from build123d import *

# Parameters (mm, degrees)
SKETCH002_R  = 1
PAD002_DEPTH = 30
PAD_DEPTH    = 6
PAD001_DEPTH = 2
SKETCH003_W  = 5
SKETCH003_H  = 5
POCKET_DEPTH = 0.5


with BuildPart() as screw_hole:
    # Sketch002 → Pad002 (new body)
    with BuildSketch(Plane.XY):
        with Locations((10, 0)):
            Circle(SKETCH002_R)
    extrude(amount=PAD002_DEPTH)


with BuildPart() as pocket:
    # Sketch → Pad (new body)
    with BuildSketch(Plane.XY):
        Polygon((0, 8.5), (8.5, 8.5), (8.5, 2.5), (11.8, 2.5), (11.8, -2.5), (8.5, -2.5), (8.5, -8.5), (0, -8.5), (0, -5.75), (5.75, -5.75), (5.75, 5.75), (0, 5.75), align=None)
    extrude(amount=PAD_DEPTH)

    # Sketch001 → Pad001 (new body)
    with BuildSketch(Plane.XY.offset(6)):
        with BuildLine():
            Line((4.9, 6.9), (6.9, 6.9))
            Line((6.9, 6.9), (6.9, 4.9))
            Line((5.678028, 4.9), (6.9, 4.9))
            ThreePointArc((5.678028, 4.9), (5.303301, 5.303301), (4.9, 5.678028))
            Line((4.9, 6.9), (4.9, 5.678028))
        make_face()
        with BuildLine():
            Line((7, -4.9), (7, -6.9))
            Line((7, -6.9), (5, -6.9))
            Line((5, -5.59017), (5, -6.9))
            ThreePointArc((5, -5.59017), (5.350155, -5.25603), (5.678028, -4.9))
            Line((5.678028, -4.9), (7, -4.9))
        make_face()
    extrude(amount=PAD001_DEPTH)

    # Cut: cut Screw Hole
    add(screw_hole.part, mode=Mode.SUBTRACT)

    # Sketch003 → Pocket (cut)
    with BuildSketch(Plane.XY.offset(6)):
        with Locations((9.9, 0)):
            Rectangle(SKETCH003_W, SKETCH003_H)
    extrude(amount=-POCKET_DEPTH, mode=Mode.SUBTRACT)


with BuildPart() as fusion:
    # Part__Mirroring: instance of Pocket
    add(pocket.part.mirror(Plane(origin=(0, 0, 0), x_dir=(0, -1, 0), z_dir=(1, 0, 0))))

    # Fusion: union Pocket
    add(pocket.part)


solid = fusion.part
The model under review builds one solid part; all positions refer to its coordinate system, in mm. A direction names the side the tool comes from. Round coordinates to 2 decimals unless told otherwise and drop trailing zeros. Loops run counter-clockwise (first coordinate to the right, second up) from the corner with the lowest first, then second, coordinate; pieces in that order, holes last. Notation, with made-up numbers: (18, 5) -> (43, 5) arc R15 ccw to (43, 22) -> close; hole circle Ø8 at (69.25, 64.5). An arc over 180 degrees is marked (long way). Answer as CSV lines item,"result".
1) Tool access review of faces 4 (the face through (-8.5, 6, 3)), 5 (the face through (8.5, 6, 3)), 6 (the face through (-6, -6.9, 7)), 7 (the face through (6, -4.9, 7)), 8 (the face through (5.75, 0, 3)): name each direction out of +Z, -Z, +X, -X, +Y, -Y from which nothing blocks a thin tool from reaching the whole face with its end or side.
Geometry results:
face 4,"+Z, -Z, -X, +Y"
face 5,"+Z, -Z, +X, +Y"
face 6,"+Z, +X, -X, -Y"
face 7,"+Z, +X, -X"
face 8,"-Z"
2) Add section D-D on y = -6.25. Write out the cut boundary in (x, z), plus the area to 3 significant figures.
Geometry results:
outline,"(-8.5, 0) -> (8.5, 0) -> (8.5, 6) -> (7, 6) -> (7, 8) -> (5, 8) -> (5, 6) -> (-5, 6) -> (-5, 8) -> (-7, 8) -> (-7, 6) -> (-8.5, 6) -> close"
area,"110 mm²"
3) To check wall thickness, follow line 1 along X through (y, z) = (0, 1.75); line 2 along Y through (x, z) = (-10, 3.7); line 3 along Y through (x, z) = (5, 1.25). State the ranges of each line that lie inside material, in increasing order. Write a range as from..to.
Geometry results:
line 1,"x = -11.8..-11, -9..-5.75, 5.75..9, 11..11.8"
line 2,"y = -2.5..-1, 1..2.5"
line 3,"y = -8.5..-5.75, 5.75..8.5"
4) For P1, Ø1.6, axis at y = 6, z = 7, coming from the -X side; P2, Ø2, axis at x = 10, y = 0.5, coming from the +Z side, all flat-tipped, find the tip position at first contact; note any pin that passes through.
Geometry results:
P1,"stops at x = -6.9"
P2,"stops at z = 5.5"
5) Add section A-A on x = 10. Write out the cut boundary in (y, z).
Geometry results:
outline,"(-2.5, 0) -> (-1, 0) -> (-1, 5.5) -> (-2.5, 5.5) -> close; (1, 0) -> (2.5, 0) -> (2.5, 5.5) -> (1, 5.5) -> close"
6) Draft analysis for pull direction Y (two halves, no side actions). For faces 1 (the face through (8.5, -5, 3)), 2 (the face through (5.43, 5.43, 6)), 3 (the face through (6, -6.9, 7)), state which applies: pulls with the +Y half, pulls with the -Y half, needs draft (parallel to the pull), parting line crosses it, or undercut.
Geometry results:
face 1,"needs draft"
face 2,"undercut"
face 3,"pulls with the -Y half"
7) Add section B-B on y = -1.25. Write out the cut boundary in (x, z).
Geometry results:
outline,"(-11.8, 0) -> (-5.75, 0) -> (-5.75, 6) -> (-7.4, 6) -> (-7.4, 5.5) -> (-11.8, 5.5) -> close; (5.75, 0) -> (11.8, 0) -> (11.8, 5.5) -> (7.4, 5.5) -> (7.4, 6) -> (5.75, 6) -> close"
8) Add section C-C on z = 5.75. Write out the cut boundary in (x, y), plus the area to 3 significant figures.
Geometry results:
outline,"(-8.5, -8.5) -> (8.5, -8.5) -> (8.5, -2.5) -> (7.4, -2.5) -> (7.4, 2.5) -> (8.5, 2.5) -> (8.5, 8.5) -> (-8.5, 8.5) -> (-8.5, 2.5) -> (-7.4, 2.5) -> (-7.4, -2.5) -> (-8.5, -2.5) -> close; hole (-5.75, -5.75) -> (5.75, -5.75) -> (5.75, 5.75) -> (-5.75, 5.75) -> close"
area,"146 mm²"
